Verification items for the finished model (mm, model axes). A direction names the side the tool comes from. Give positions to 0.01 mm unless a question says otherwise; leave off trailing zeros. Loops run counter-clockwise (first coordinate to the right, second up) from the corner with the lowest first, then second, coordinate; pieces in that order, holes last. Notation, with made-up numbers: M 29.5,-4 L 47.5,-4 A20 cw 47.5,1 Z; hole C 76.25,-3.5 d8. An arc over 180 degrees is marked long. Answer in a Markdown table with one row per item.
Autodesk Inventor part; units mm, degrees
ref_plane "YZ Plane" through (0, 0, 0) normal (1, 0, 0) x (0, 1, 0)
ref_plane "XZ Plane" through (0, 0, 0) normal (0, 1, 0) x (-1, 0, 0)
ref_plane "XY Plane" through (0, 0, 0) normal (0, 0, 1) x (1, 0, 0)
sketch "Sketch1" plane through (0, 0, 0) normal (0, 0, 1) x (1, 0, 0)
  line L0 (0, 0) -> (-75, 0)
  line L1 (-75, 0) -> (-75, 180)
  line L2 (-75, 180) -> (0, 180)
  line L3 (0, 180) -> (0, 0)
  line L4 (-65, 170) -> (-10, 170)
  line L5 (-10, 10) -> (-65, 10)
  line L6 (-65, 10) -> (-65, 85)
  line L7 (-65, 95) -> (-65, 170)
  line L8 (-10, 170) -> (-10, 95)
  line L9 (-10, 85) -> (-10, 10)
  line L10 (-65, 85) -> (-65, 95)
  line L11 (-10, 95) -> (-10, 85)
  point P0 (-65, 90)
  point P1 (-10, 90)
  dimension "d35" = 75
  dimension "d36" = 180
  dimension "d37" = 55
  dimension "d38" = 160
extrude "Extrusion7" add sketch "Sketch1" along normal blind 70
sketch "Sketch6" plane through (0, 0, 0) normal (1, 0, 0) x (0, 0, -1)
  line L0 (-10, 62.5) -> (-65, 62.5)
  line L1 (-65, 62.5) -> (-65, 117.5)
  line L2 (-65, 117.5) -> (-10, 117.5)
  line L3 (-10, 117.5) -> (-10, 62.5)
  dimension "d67" = 55
  dimension "d68" = 55
extrude "Extrusion10" cut sketch "Sketch6" against normal blind 2
sketch "Sketch7" plane through (-75, 0, 0) normal (-1, 0, 0) x (0, 0, 1)
  line L0 (10, 62.5) -> (65, 62.5)
  line L1 (10, 62.5) -> (65, 62.5)
  line L2 (65, 62.5) -> (65, 117.5)
  line L3 (65, 117.5) -> (10, 117.5)
  line L4 (10, 117.5) -> (10, 62.5)
  point P0 (0, 0)
  dimension "d71" = 55
  dimension "d72" = 55
extrude "Extrusion11" cut sketch "Sketch7" against normal blind 2
sketch "Sketch8" plane through (-75, 0, 0) normal (0, -1, 0) x (1, 0, 0)
  line L0 (10, 10) -> (65, 10)
  line L1 (65, 10) -> (65, 65)
  line L2 (65, 65) -> (10, 65)
  line L3 (10, 65) -> (10, 10)
  point P0 (75, 0)
  dimension "d75" = 55
  dimension "d76" = 55
extrude "Extrusion12" cut sketch "Sketch8" against normal blind 2
sketch "Sketch9" plane through (-75, 180, 0) normal (0, 1, 0) x (1, 0, 0)
  line L0 (10, -10) -> (65, -10)
  line L1 (65, -10) -> (65, -65)
  line L2 (65, -65) -> (10, -65)
  line L3 (10, -65) -> (10, -10)
  point P0 (75, 0)
  dimension "d79" = 55
  dimension "d80" = 55
extrude "Extrusion13" cut sketch "Sketch9" against normal blind 2
sketch "Sketch10" plane through (-75, 0, 0) normal (0, -1, 0) x (1, 0, 0)
  line L0 (74, 1) -> (63.4, 1)
  line L1 (63.4, 1) -> (63.4, 6.6)
  line L2 (63.4, 6.6) -> (74, 6.6)
  line L3 (74, 6.6) -> (74, 1)
  line L4 (1, 1) -> (11.6, 1)
  line L5 (11.6, 1) -> (11.6, 6.6)
  line L6 (11.6, 6.6) -> (1, 6.6)
  line L7 (1, 6.6) -> (1, 1)
  point P0 (75, 0)
  dimension "d83" = 10.6
  dimension "d84" = 5.6
  dimension "d85" = 10.6
  dimension "d86" = 5.6
extrude "Extrusion14" cut sketch "Sketch10" against normal blind 5
sketch "Sketch11" plane through (-75, 180, 0) normal (0, 1, 0) x (1, 0, 0)
  line L0 (1, -1) -> (11.6, -1)
  line L1 (11.6, -1) -> (11.6, -6.6)
  line L2 (11.6, -6.6) -> (1, -6.6)
  line L3 (1, -6.6) -> (1, -1)
  line L4 (74, -1) -> (63.4, -1)
  line L5 (63.4, -1) -> (63.4, -6.6)
  line L6 (63.4, -6.6) -> (74, -6.6)
  line L7 (74, -6.6) -> (74, -1)
  point P0 (75, 0)
  dimension "d89" = 10.6
  dimension "d90" = 5.6
  dimension "d91" = 10.6
  dimension "d92" = 5.6
extrude "Extrusion15" cut sketch "Sketch11" against normal blind 5
properties part number "Shoulder_Cube_TestFit_V1"
Item 1: Sectioned sample at B-B (x = -25.5). Record the cut outline in (y, z), and give its area (3 significant figures).
Reported:
| item | result |
|---|---|
| outline | M 0,0 L 10,0 L 10,70 L 0,70 L 0,65 L 2,65 L 2,10 L 0,10 Z; M 170,0 L 180,0 L 180,10 L 178,10 L 178,65 L 180,65 L 180,70 L 170,70 Z |
| area | 1,180 mm^2 |
Item 2: Sectioned sample at D-D (y = 29.5). Record the cut outline in (x, z).
Reported:
| item | result |
|---|---|
| outline | M -75,0 L -65,0 L -65,70 L -75,70 Z; M -10,0 L 0,0 L 0,70 L -10,70 Z |
Item 3: Scan lines: L1, parallel to Y at x = -46.5, z = 64; L2, parallel to X at y = 83.5, z = 50.5; L3, parallel to X at y = 31.5, z = 25. Record each from-to range of solid material in increasing order. Write a range as [from, to].
Reported:
| item | result |
|---|---|
| L1 | y = [2, 10], [170, 178] |
| L2 | x = [-73, -65], [-10, -2] |
| L3 | x = [-75, -65], [-10, 0] |
Item 4: Go/stop test with flat-tipped pins: pin 1 (16.5 mm diameter, centred on x = -32.5, z = 45.5, fed in from -Y); pin 2 (1.5 mm diameter, centred on x = -52, z = 36.5, fed in from +Y); pin 3 (4 mm diameter, centred on y = 66, z = 20.5, fed in from -X). Record where each tip stops, or that it passes through.
Reported:
| item | result |
|---|---|
| pin 1 | stops at y = 2 |
| pin 2 | stops at y = 178 |
| pin 3 | stops at x = -73 |
Item 5: Sectioned sample at A-A (y = 105). Record the cut outline in (x, z), and give its area (3 significant figures).
Reported:
| item | result |
|---|---|
| outline | M -75,0 L -65,0 L -65,70 L -75,70 L -75,65 L -73,65 L -73,10 L -75,10 Z; M -10,0 L 0,0 L 0,10 L -2,10 L -2,65 L 0,65 L 0,70 L -10,70 Z |
| area | 1,180 mm^2 |
Item 6: Release check for a two-part mould opening along Z. For faces 4 (the flat face through (-37, 10, 35)), 5 (the flat face through (-69, 178, 1)) record: released by +Z, released by -Z, zero draft, split by the parting line, or undercut.
Reported:
| item | result |
|---|---|
| face 4 | zero draft |
| face 5 | undercut |
Item 7: Tool access check on faces 1 (the flat face through (-11.6, 2, 4)), 2 (the flat face through (-65, 89, 35)), 3 (the flat face through (-6, 175, 4)). Record the directions out of +Z, -Z, +X, -X, +Y, -Y that give a thin tool (end or side, any length) a straight path to the whole face; none if there is none.
Reported:
| item | result |
|---|---|
| face 1 | -Y |
| face 2 | +Z, -Z |
| face 3 | +Y |
Item 8: Sectioned sample at C-C (z = 34). Record the cut outline in (x, y).
Reported:
| item | result |
|---|---|
| outline | M -75,0 L -65,0 L -65,2 L -10,2 L -10,0 L 0,0 L 0,62.5 L -2,62.5 L -2,117.5 L 0,117.5 L 0,180 L -10,180 L -10,178 L -65,178 L -65,180 L -75,180 L -75,117.5 L -73,117.5 L -73,62.5 L -75,62.5 Z; hole M -65,10 L -10,10 L -10,170 L -65,170 Z |
